For this review, use the dimensioned drawing (mm, ordinates from the lowest corner) and the shaded views. A direction names the side the tool comes from. Coordinates: 2 decimals unless noted, no trailing zeros. Loops run counter-clockwise (first coordinate to the right, second up) from the corner with the lowest first, then second, coordinate; pieces in that order, holes last. Notation, with made-up numbers: (-18.75, 18.5) - (13.25, 18.5) arc R23 cw to (13.25, 33.5) - close; hole circle Ø9 at (-7.75, 68.5). An arc over 180 degrees is marked (long way). Answer in a Markdown table with one row per item. Add a question column.
(1) We need section D-D on z = 4.5. Write out the cut boundary in (x, y), plus the area to 3 significant figures.
(2) Machinability: for the marked faces 3 and 4, which of the approach directions +Z, -Z, +X, -X, +Y, -Y give a long, thin tool a straight path to every point of the face, cutting with its end or side? Answer none if there is none.
(3) For line 1 along X through (y, z) = (3.1, 8); line 2 along Z through (x, y) = (20, 1); line 3 along X through (y, z) = (2, 20), list the stretches that pass through material, from the lowest coordinate up.
(4) For P1, Ø1.2, axis at y = 3.5, z = 23.5, coming from the -X side, flat-tipped, find the tip position at first contact; note if it passes through.
(5) We need section A-A on z = 20. Write out the cut boundary in (x, y), plus the area to 3 significant figures.
(6) Mouldability with a two-part tool opening along X and no side actions: class the marked faces 1 and 2 as +X half, -X half, draft (parallel to the pull), parting line (faces both ways), or undercut.
(7) We need section B-B on x = 20. Write out the cut boundary in (y, z).
(8) We need section C-C on y = 2.25. Write out the cut boundary in (x, z).
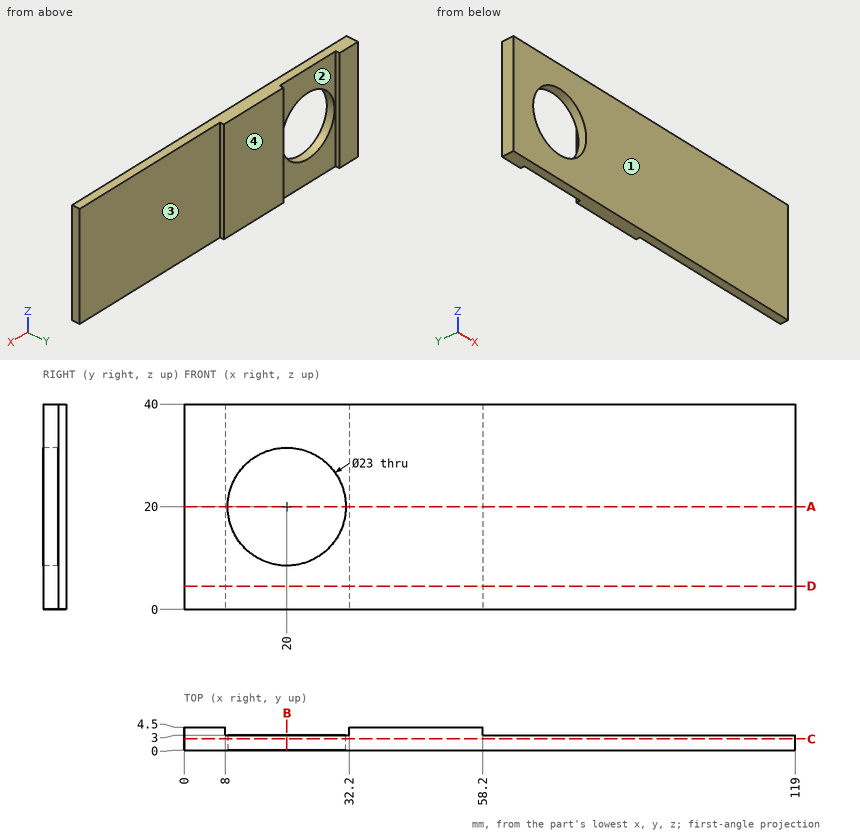
Outcome:
| question | item | result |
|---|---|---|
| 1 | outline | (0, 0) - (119, 0) - (119, 3) - (58.2, 3) - (58.2, 4.5) - (32.2, 4.5) - (32.2, 3) - (8, 3) - (8, 4.5) - (0, 4.5) - close |
| 1 | area | 408 mm² |
| 2 | face 3 | +Z, -Z, +X, +Y |
| 2 | face 4 | +Z, -Z, +X, -X, +Y |
| 3 | line 1 | 0 to 8, 32.2 to 58.2 |
| 3 | line 2 | 0 to 8.5, 31.5 to 40 |
| 3 | line 3 | 0 to 8.5, 31.5 to 119 |
| 4 | P1 | x = 0 |
| 5 | outline | (0, 0) - (8.5, 0) - (8.5, 3) - (8, 3) - (8, 4.5) - (0, 4.5) - close; (31.5, 0) - (119, 0) - (119, 3) - (58.2, 3) - (58.2, 4.5) - (32.2, 4.5) - (32.2, 3) - (31.5, 3) - close |
| 5 | area | 339 mm² |
| 6 | face 1 | draft |
| 6 | face 2 | undercut |
| 7 | outline | (0, 0) - (3, 0) - (3, 8.5) - (0, 8.5) - close; (0, 31.5) - (3, 31.5) - (3, 40) - (0, 40) - close |
| 8 | outline | (0, 0) - (119, 0) - (119, 40) - (0, 40) - close; hole circle Ø23 at (20, 20) |
